Geometry: final body of the model. Coordinates: model frame, mm. A direction names the side the tool comes from. Give positions to 0.01 mm unless a question says otherwise; leave off trailing zeros. Loops run counter-clockwise (first coordinate to the right, second up) from the corner with the lowest first, then second, coordinate; pieces in that order, holes last. Notation, with made-up numbers: (53.5, 46) - (78.5, 46) arc R23 cw to (78.5, 80) - close; hole circle Ø5 at (-18, 3.5). An arc over 180 degrees is marked (long way). Answer in a Markdown table with one row per item.
Autodesk Inventor part; units mm, degrees
ref_plane "YZ Plane" through (0, 0, 0) normal (1, 0, 0) x (0, 1, 0)
ref_plane "XZ Plane" through (0, 0, 0) normal (0, 1, 0) x (-1, 0, 0)
ref_plane "XY Plane" through (0, 0, 0) normal (0, 0, 1) x (1, 0, 0)
sketch "Sketch1" plane through (0, 0, 0) normal (0, 0, 1) x (1, 0, 0)
  line L0 (66.7253, 90.1264) -> (-18.9997, 90.1264)
  line L1 (-18.9997, 90.1264) -> (-18.9997, 52.0264)
  line L2 (-18.9997, 52.0264) -> (66.7253, 52.0264)
  line L3 (66.7253, 52.0264) -> (66.7253, 90.1264)
  line L4 (66.7253, 78.1884) -> (-18.9997, 78.1884)
  line L5 (-18.9997, 78.1884) -> (-18.9997, 76.5584)
  line L6 (-18.9997, 76.5584) -> (66.7253, 76.5584)
  line L7 (66.7253, 76.5584) -> (66.7253, 78.1884)
  line L8 (55.9303, 78.1884) -> (55.9303, 76.5584)
  line L9 (-11.3797, 76.5584) -> (-11.3797, 78.1884)
  point P0 (0, 0)
  dimension "d0" = 38.1
  dimension "d1" = 85.725
  dimension "d2" = 1.63
  dimension "d3" = 11.938
  dimension "d6" = 67.31
  dimension "d7" = 7.62
extrude "Extrusion1" add sketch "Sketch1" along normal blind 3.175 contours L3 L4 L1 L0 | L3 L6 L8 L4 | L4 L9 L6 L1 | L3 L2 L1 L6
sketch "Sketch2" plane through (0, 0, 0) normal (0, 0, -1) x (-1, 0, 0)
  line L0 (-55.9303, 78.1884) -> (11.3797, 78.1884)
  line L1 (11.3797, 78.1884) -> (11.3797, 76.5584)
  line L2 (-6.2385, 84.1043) -> (3.2865, 84.1043)
  line L3 (3.2865, 84.1043) -> (3.2865, 74.5793)
  line L4 (3.2865, 74.5793) -> (-6.2385, 74.5793)
  line L5 (-6.2385, 74.5793) -> (-6.2385, 84.1043)
  line L6 (-47.533, 84.1043) -> (-38.008, 84.1043)
  line L7 (-38.008, 84.1043) -> (-38.008, 74.5865)
  line L8 (-38.008, 74.5865) -> (-47.533, 74.5865)
  line L9 (-47.533, 74.5865) -> (-47.533, 84.1043)
  line L10 (18.9997, 52.0264) -> (-66.7253, 52.0264)
  line L11 (-34.9753, 52.0264) -> (3.1247, 52.0264)
  line L12 (3.1247, 52.0264) -> (3.1247, 58.3764)
  line L13 (3.1247, 58.3764) -> (-34.9753, 58.3764)
  line L14 (-34.9753, 58.3764) -> (-34.9753, 52.0264)
  line L15 (-66.7253, 52.0264) -> (-66.7253, 90.1264)
  line L16 (-66.7253, 90.1264) -> (18.9997, 90.1264)
  line L17 (-34.9753, 90.1264) -> (-22.2753, 90.1264)
  line L18 (-22.2753, 90.1264) -> (-22.2753, 87.5864)
  line L19 (-22.2753, 87.5864) -> (-34.9753, 87.5864)
  line L20 (-34.9753, 87.5864) -> (-34.9753, 90.1264)
  point P0 (0, 0)
  dimension "d8" = 9.525
  dimension "d9" = 9.5177
  dimension "d10" = 9.525
  dimension "d11" = 9.525
  dimension "d12" = 31.7695
  dimension "d13" = 5.9159
  dimension "d14" = 8.0932
  dimension "d17" = 6.35
  dimension "d18" = 38.1
  dimension "d20" = 2.54
  dimension "d21" = 12.7
  dimension "d22" = 31.75
  dimension "d23" = 31.75
extrude "Extrusion2" cut sketch "Sketch2" against normal blind 3.175
properties part number "RearBulkhead"
Q1. Reachability of faces 1 (the flat face through (34.975, 89, 2)), 2 (the flat face through (2, 84.104, 2)), 3 (the flat face through (-3.125, 55, 2)) from +Z, -Z, +X, -X, +Y, -Y: full face, straight path, thin tool, end or side. Return the list, or none.
Check values:
| item | result |
|---|---|
| face 1 | +Z, -Z, +Y |
| face 2 | +Z, -Z |
| face 3 | +Z, -Z, -Y |
Q2. Cut plane B-B (x = 29). Output: boundary loops of the cut face in (y, z) (3 decimals), and give its area (3 significant figures).
Check values:
| item | result |
|---|---|
| outline | (58.376, 0) - (76.558, 0) - (76.558, 3.175) - (58.376, 3.175) - close; (78.188, 0) - (87.586, 0) - (87.586, 3.175) - (78.188, 3.175) - close |
| area | 87.6 mm² |
Q3. Draft query along X for faces 4 (the flat face through (66.725, 71, 2)), 5 (the flat face through (22, 78.188, 2)), 6 (the flat face through (51, 52.026, 2)). Return one class per face: pulls with the +X half, pulls with the -X half, needs draft (parallel to the pull), parting line crosses it, or undercut.
Check values:
| item | result |
|---|---|
| face 4 | pulls with the +X half |
| face 5 | undercut |
| face 6 | needs draft |
Q4. Material intervals for line 1 along X through (y, z) = (79, 2.15); line 2 along Y through (x, z) = (-10.5, 2.85); line 3 along X through (y, z) = (57, 0.3), sorted ascending.
Check values:
| item | result |
|---|---|
| line 1 | -19 to -3.29, 6.24 to 38.01, 47.53 to 66.73 |
| line 2 | 52.03 to 76.56, 78.19 to 90.13 |
| line 3 | -19 to -3.12, 34.98 to 66.73 |
Q5. First-contact query: pin 1 (5 mm diameter, centred on x = 32.5, y = 76, fed in from -Z); pin 2 (1.6 mm diameter, centred on x = 20.5, z = 2, fed in from -Y). Flat tips, straight axial feed; report the tip coordinate or a pass-through.
Check values:
| item | result |
|---|---|
| pin 1 | z = 0 |
| pin 2 | y = 58.38 |
Q6. Cut plane A-A (y = 56.5). Output: boundary loops of the cut face in (x, z) (3 decimals), and give its area (3 significant figures).
Check values:
| item | result |
|---|---|
| outline | (-19, 0) - (-3.125, 0) - (-3.125, 3.175) - (-19, 3.175) - close; (34.975, 0) - (66.725, 0) - (66.725, 3.175) - (34.975, 3.175) - close |
| area | 151 mm² |
